```python
from build123d import *

# Parameters (mm, degrees)
SKETCH009_W      = 35.3624
SKETCH009_H      = 77.7328
PAD004_DEPTH     = 2.5
SKETCH010_R      = 2.25
PAD005_DEPTH     = 6.9
HOLE_D           = 2.7
HOLE_CSINK_D     = 4.5
HOLE_CSINK_ANGLE = 90


with BuildPart() as part:
    # Sketch009 (on CopyDatumPlane) → Pad004 (new body)
    with BuildSketch(Plane.XY.offset(8.5)):
        with Locations((14.6812, 25.8664)):
            Rectangle(SKETCH009_W, SKETCH009_H)
    extrude(amount=PAD004_DEPTH)

    # Sketch010 (on CopyDatumPlane) → Pad005 (join)
    with BuildSketch(Plane.XY.offset(8.5)):
        with Locations((2.1844, 57.038)):
            Circle(SKETCH010_R)
        with Locations((27.178, 57.038)):
            Circle(SKETCH010_R)
        with Locations((27.178, 2.174)):
            Circle(SKETCH010_R)
        with Locations((2.1844, 2.174)):
            Circle(SKETCH010_R)
    extrude(amount=-PAD005_DEPTH)

    # Hole (through all)
    with Locations(Plane.XY.offset(11)):
        with Locations((-0.5, 62.2328), (29.8624, 62.2328), (29.8624, -10.5), (-0.5, -10.5)):
            CounterSinkHole(HOLE_D / 2, HOLE_CSINK_D / 2, counter_sink_angle=HOLE_CSINK_ANGLE)


solid = part.part
```
Input: part model. Units: mm. Frame: model coordinates. A direction names the side the tool comes from. Coordinates: 2 decimals unless noted, no trailing zeros. Write each loop counter-clockwise with the first axis right and the second up, starting at its lowest first coordinate (ties: lowest second). Pieces come first, ordered by that corner, then holes. Notation, with made-up numbers: (57, 81.25) -> (85, 81.25) arc R30 ccw to (85, 114.25) -> close; hole circle Ø10 at (85.25, 36). An arc over 180 degrees is marked (long way). Write each question's results on one line, items separated by ' | '.
Item 1: Pin query (flat end, axial travel): pin 1 Ø1 at (x, y) = (3, 42.5) entering from -Z; pin 2 Ø3 at (x, y) = (29.86, -10.5) entering from +Z; pin 3 Ø3 at (x, z) = (28.5, 5.5) entering from -Y. Return the tip coordinate at first contact, or that it passes through.
Conclusion:
pin 1: stops at z = 8.5 | pin 2: stops at z = 10.25 | pin 3: stops at y = -0.08
Item 2: Material intervals for probe 1 along X at (y, z) = (-10.5, 9.2); probe 2 along Z at (x, y) = (8.5, -9); probe 3 along Y at (x, z) = (25.5, 3.25), sorted ascending.
Conclusion:
probe 1: x = -3 to -1.85, 0.85 to 28.51, 31.21 to 32.36 | probe 2: z = 8.5 to 11 | probe 3: y = 0.68 to 3.67, 55.54 to 58.54
Item 3: Section query A-A on y = -10.5. Return loops of the section in (x, z).
Conclusion:
outline: (-3, 8.5) -> (-1.85, 8.5) -> (-1.85, 10.1) -> (-2.75, 11) -> (-3, 11) -> close; (0.85, 8.5) -> (28.51, 8.5) -> (28.51, 10.1) -> (27.61, 11) -> (1.75, 11) -> (0.85, 10.1) -> close; (31.21, 8.5) -> (32.36, 8.5) -> (32.36, 11) -> (32.11, 11) -> (31.21, 10.1) -> close
Item 4: Section query C-C on z = 3.5. Return loops of the section in (x, y).
Conclusion:
outline: circle Ø4.5 at (2.18, 2.17); circle Ø4.5 at (2.18, 57.04); circle Ø4.5 at (27.18, 2.17); circle Ø4.5 at (27.18, 57.04)
Item 5: Mould query, pull axis X, two halves, no side actions, for faces 1 (the flat face through (14, 26, 11)), 2 (the cylindrical face through (28.575, -10.094, 9.289)), 3 (the flat face through (-3, 25, 10)), 4 (the cylindrical face through (-0.207, 60.915, 9.289)). Classes: +X half, -X half, draft (parallel to the pull), parting line (faces both ways), or undercut.
Conclusion:
face 1: draft | face 2: undercut | face 3: -X half | face 4: undercut
Item 6: Section query D-D on y = 31.5. Return loops of the section in (x, z), plus the area to 3 significant figures.
Conclusion:
outline: (-3, 8.5) -> (32.36, 8.5) -> (32.36, 11) -> (-3, 11) -> close | area: 88.4 mm^2
Item 7: Set-up query: faces 5 (the flat face through (27, 57, 1.6)), 6 (the cylindrical face through (3.223, 0.178, 5.098)). Return all of +Z, -Z, +X, -X, +Y, -Y with unobstructed straight access to the full face (end or side cutting, diameter ignored); none if empty.
Conclusion:
face 5: -Z, +X, -X, +Y, -Y | face 6: -Z
Item 8: Section query B-B on x = 12. Return loops of the section in (y, z).
Conclusion:
outline: (-13, 8.5) -> (64.73, 8.5) -> (64.73, 11) -> (-13, 11) -> close
